Verification items for this drawing (mm, ordinates from the low corner). A direction names the side the tool comes from. Round coordinates to 2 decimals unless told otherwise and drop trailing zeros. Loops run counter-clockwise (first coordinate to the right, second up) from the corner with the lowest first, then second, coordinate; pieces in that order, holes last. Notation, with made-up numbers: M 55.5,27 L 96.5,27 A25 ccw 96.5,63 Z; hole C 41,63.5 d5. An arc over 180 degrees is marked long. One line per item, written item: value.
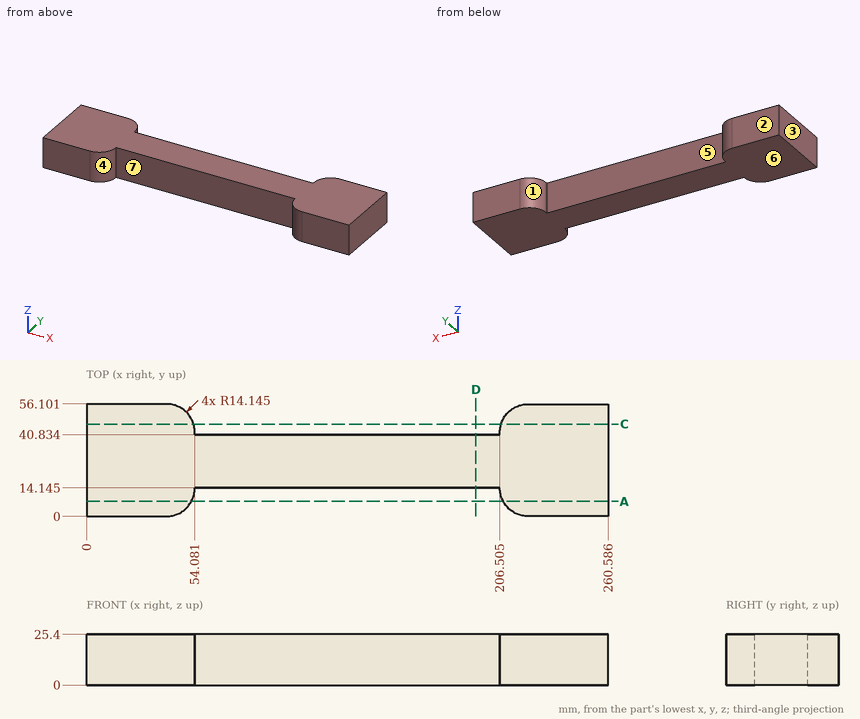
(1) Tool access check on the marked faces 5, 6 and 7. Record the directions out of +Z, -Z, +X, -X, +Y, -Y that give a thin tool (end or side, any length) a straight path to the whole face; none if there is none.
Completed:
face 5: +Z, -Z, +Y
face 6: -Z, +X, -X, +Y, -Y
face 7: +Z, -Z, -Y
(2) Sectioned sample at C-C on y = 46. Enter the section's corners in (x, z) (1 decimal).
Completed:
outline: M 0,0 L 53.5,0 L 53.5,25.4 L 0,25.4 Z; M 207.1,0 L 260.6,0 L 260.6,25.4 L 207.1,25.4 Z
(3) Mould release check, pull along X, two halves, no side actions. Record for the marked faces 1, 2, 3 and 4: +X half, -X half, draft (parallel to the pull), parting line (faces both ways), or undercut.
Completed:
face 1: undercut
face 2: draft
face 3: -X half
face 4: undercut
(4) Depth check by flat-ended pin: pin 1 Ø4 at (x, y) = (118.5, 11) entering from -Z; pin 2 Ø8 at (x, z) = (207, 11.5) entering from -Y; pin 3 Ø7.5 at (x, z) = (166.5, 16.5) entering from +Y. Enter the tip coordinate at first touch or a pass-through.
Completed:
pin 1: passes through
pin 2: stops at y = 3.8
pin 3: stops at y = 40.83
(5) Thickness scan on L1, parallel to X at y = 12, z = 19.5 (1 decimal); L2, parallel to Y at x = 169.5, z = 12.5 (1 decimal); L3, parallel to X at y = 48.5, z = 11.25 (1 decimal). Record the ranges inside material, lowest first. Write a range as from..to.
Completed:
L1: x = 0..53.9, 206.7..260.6
L2: y = 14.1..40.8
L3: x = 0..52.5, 208.1..260.6
(6) Sectioned sample at D-D on x = 194.5. Enter the section's corners in (y, z) (1 decimal), and give its area (3 significant figures).
Completed:
outline: M 14.1,0 L 40.8,0 L 40.8,25.4 L 14.1,25.4 Z
area: 678 mm^2
(7) Sectioned sample at A-A on y = 7.5. Enter the section's corners in (x, z) (1 decimal), and give its area (3 significant figures).
Completed:
outline: M 0,0 L 52.4,0 L 52.4,25.4 L 0,25.4 Z; M 208.2,0 L 260.6,0 L 260.6,25.4 L 208.2,25.4 Z
area: 2,660 mm^2
